CAD build for the part. Positions are in the model's coordinates, mm. Face numbers are marked on the shaded views. Give positions to 0.01 mm unless a question says otherwise; leave off trailing zeros. Order: outer loops, then holes, each group sorted by start corner. A loop starts at its lowest first (then second) coordinate and runs counter-clockwise, first axis right, second up.
Item 1: Two-plate mould, pull along X, no slides. Class the marked faces 1, 2 and 3: released by +X, released by -X, zero draft, split by the parting line, or undercut.
Item 2: Band-saw the part on A-A on z = 0. Give the cut face in (x, y), plus the area to 3 significant figures.
Item 3: Band-saw the part on C-C on y = -67. Give the cut face in (x, z), plus the area to 3 significant figures.
Item 4: Band-saw the part on D-D on z = 50. Give the cut face in (x, y).
Item 5: Wall check: L1, parallel to X at y = -5, z = 106; L2, parallel to Z at x = 7.5, y = 0; L3, parallel to Y at x = 15, z = 0. Give the ranges that are in metal, low to high.
Item 6: Flat gauge pins, fed straight in: P1, Ø23, axis at y = 0, z = 0, coming from the -X side; P2, Ø2, axis at x = 5.5, z = 21, coming from the -Y side; P3, Ø2, axis at x = 10.5, y = 30.5, coming from the -Z side; P4, Ø1, axis at x = -14.5, z = 4, coming from the +Y side. Where does each tip first touch, or does it go through?
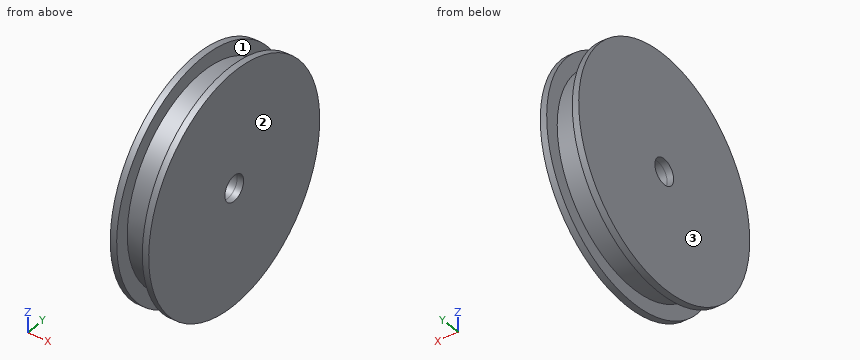
Autodesk Inventor part; units mm, degrees
ref_plane "XZ Plane" through (0, 0, 0) normal (0, 1, 0) x (-1, 0, 0)
ref_plane "XY Plane" through (0, 0, 0) normal (0, 0, 1) x (1, 0, 0)
sketch "Sketch1" plane through (0, 0, 0) normal (1, 0, 0) x (0, 1, 0)
  circle A0 centre (0, 0) radius 101.6
  circle A1 centre (0, 0) radius 12.7
  dimension "d0" = 203.2
  dimension "d1" = 25.4
extrude "Extrusion1" add sketch "Sketch1" along normal mid plane 25.4
sketch "Sketch3" plane through (12.7, 0, 0) normal (1, 0, 0) x (0, 0, -1)
  circle A0 centre (0, 0) radius 12.7
  circle A1 centre (0, 0) radius 115.8875
  dimension "d7" = 25.4
  dimension "d8" = 231.775
extrude "Extrusion3" add sketch "Sketch3" along normal blind 6.35
mirror "Mirror1" about plane through (0, 0, 0) normal (1, 0, 0) of "Extrusion3"
properties part number "Wheel" material "Wood (Birch)"
The answers:
1. face 1: undercut
1. face 2: released by +X
1. face 3: released by -X
2. outline: (-19.05, -115.89) - (-12.7, -115.89) - (-12.7, -101.6) - (12.7, -101.6) - (12.7, -115.89) - (19.05, -115.89) - (19.05, -12.7) - (-19.05, -12.7) - close; (-19.05, 12.7) - (19.05, 12.7) - (19.05, 115.89) - (12.7, 115.89) - (12.7, 101.6) - (-12.7, 101.6) - (-12.7, 115.89) - (-19.05, 115.89) - close
2. area: 7,140 mm2
3. outline: (-19.05, -94.56) - (-12.7, -94.56) - (-12.7, -76.38) - (12.7, -76.38) - (12.7, -94.56) - (19.05, -94.56) - (19.05, 94.56) - (12.7, 94.56) - (12.7, 76.38) - (-12.7, 76.38) - (-12.7, 94.56) - (-19.05, 94.56) - close
3. area: 6,280 mm2
4. outline: (-19.05, -104.55) - (-12.7, -104.55) - (-12.7, -88.45) - (12.7, -88.45) - (12.7, -104.55) - (19.05, -104.55) - (19.05, 104.55) - (12.7, 104.55) - (12.7, 88.45) - (-12.7, 88.45) - (-12.7, 104.55) - (-19.05, 104.55) - close
5. L1: x = -19.05 to -12.7, 12.7 to 19.05
5. L2: z = -101.6 to -12.7, 12.7 to 101.6
5. L3: y = -115.89 to -12.7, 12.7 to 115.89
6. P1: passes through
6. P2: stops at y = -99.61
6. P3: stops at z = -97.22
6. P4: stops at y = 115.83
